Design review of the part built by this model. Coordinates are the model's own, in mm. A direction names the side the tool comes from. Give positions to 0.01 mm unless a question says otherwise; leave off trailing zeros. Loops run counter-clockwise (first coordinate to the right, second up) from the corner with the lowest first, then second, coordinate; pieces in that order, holes last. Notation, with made-up numbers: M 16.5,1.25 L 21.5,1.25 A7 cw 21.5,12.25 Z; hole C 81.25,71.25 d1. An arc over 180 degrees is marked long. Use a Markdown table: item, result. Add a question column.
(1) Draft analysis for pull direction Z (two halves, no side actions). For faces 6 (the face through (-7.5, -19.1, 19.2)), 7 (the face through (-1.404, -15.612, 15.676)), 8 (the face through (-5, -0.1, 20.5)), state which applies: pulls with the +Z half, pulls with the -Z half, needs draft (parallel to the pull), parting line crosses it, or undercut.
(2) Add section D-D, the plane z = 12. Give the boundary of the cut face in (x, y).
(3) Add section C-C, the plane x = 2. Give the boundary of the cut face in (y, z), then the cut area to 3 significant figures.
(4) Insertion check: pin 1 Ø4 at (y, z) = (15.5, 15.5) entering from -X; pin 2 Ø8 at (x, y) = (0, 7) entering from -Z; pin 3 Ø8 at (x, z) = (-0.5, -4.5) entering from +Y. Each pin has a flat end and moves straight along its axis. Give the tip position at first contact, or say it passes through.
(5) For faces 1 (the face through (0, -20.15, 0)), 2 (the face through (8, 0, 21.15)), 3 (the face through (0.07, -18.467, 18.419)), 4 (the face through (8, 0, -21.15)), 5 (the face through (-5.94, 15.24, 14.33)), list the 3-axis set-ups (+Z, -Z, +X, -X, +Y, -Y) from which the entire face can be reached by the end or side of a thin tool; tool diameter is ignored.
(6) For probe 1 along Y at (x, z) = (-4.25, -15.5); probe 2 along Z at (x, y) = (-6.75, 15.5), list the stretches that pass through material, from the lowest coordinate up.
(7) Add section A-A, the plane y = 0. Give the boundary of the cut face in (x, z).
```python
from build123d import *

# Parameters (mm, degrees)
F0_W     = 42.3
F0_H     = 42.3
F1_DEPTH = 10
F2_SIZE  = 4
F3_W     = 43
F3_H     = 43
F4_DEPTH = 5
F5_R     = 2.5
F6_DEPTH = 20
F8_D     = 2.4
F8_DEPTH = 8
F8_TIP   = 0.7210327428


with BuildPart() as f1:
    # F0 (on Right) → F1 (new body, symmetric)
    with BuildSketch(Plane.YZ):
        Rectangle(F0_W, F0_H)
    extrude(amount=F1_DEPTH, both=True)

    # F2
    f2_edges = [f1.edges().sort_by_distance(p)[0] for p in [
        (0, -21.15, 21.15),
        (0, 21.15, 21.15),
        (0, -21.15, -21.15),
        (0, 21.15, -21.15),
    ]]
    chamfer(f2_edges, length=F2_SIZE)

    # F3 (on Right) → F4 (cut, symmetric)
    with BuildSketch(Plane.YZ):
        Rectangle(F3_W, F3_H)
        Polygon((-16.7357864376, -20.15), (-20.15, -16.7357864376), (-20.15, 16.7357864376), (-16.7357864376, 20.15), (16.7357864376, 20.15), (20.15, 16.7357864376), (20.15, -16.7357864376), (16.7357864376, -20.15), align=None, mode=Mode.SUBTRACT)
    extrude(amount=F4_DEPTH, both=True, mode=Mode.SUBTRACT)

    # F5 (on face) → F6 (join)
    with BuildSketch(Plane(origin=(-10, 0, 0), x_dir=(0, -1, 0), z_dir=(-1, 0, 0))):
        Circle(F5_R)
    extrude(amount=F6_DEPTH)

    # F8
    with Locations(Plane(origin=(-10, 0, 0), x_dir=(0, -1, 0), z_dir=(-1, 0, 0))):
        with Locations((-15.5, 15.5), (15.5, 15.5), (-15.5, -15.5), (15.5, -15.5)):
            Hole(F8_D / 2, depth=F8_DEPTH)
            with Locations((0, 0, -(F8_DEPTH + F8_TIP / 2))):  # 118° drill point
                Cone(0, F8_D / 2, F8_TIP, mode=Mode.SUBTRACT)


solid = f1.part
```
Established:
| question | item | result |
|---|---|---|
| 1 | face 6 | pulls with the +Z half |
| 1 | face 7 | undercut |
| 1 | face 8 | needs draft |
| 2 | outline | M -10,-21.15 L -5,-21.15 L -5,-20.15 L 5,-20.15 L 5,-21.15 L 10,-21.15 L 10,21.15 L 5,21.15 L 5,20.15 L -5,20.15 L -5,21.15 L -10,21.15 Z |
| 3 | outline | M -20.15,-16.74 L -16.74,-20.15 L 16.74,-20.15 L 20.15,-16.74 L 20.15,16.74 L 16.74,20.15 L -16.74,20.15 L -20.15,16.74 Z |
| 3 | area | 1,600 mm^2 |
| 4 | pin 1 | x = -10 |
| 4 | pin 2 | z = -20.15 |
| 4 | pin 3 | y = 20.15 |
| 5 | face 1 | +Z, -Z, -Y |
| 5 | face 2 | +Z, +X, -X, +Y, -Y |
| 5 | face 3 | +Z, -Y |
| 5 | face 4 | -Z, +X, -X, +Y, -Y |
| 5 | face 5 | -X |
| 6 | probe 1 | -20.15 to -16.7, -14.3 to 14.3, 16.7 to 20.15 |
| 6 | probe 2 | -21.15 to -16.7, -14.3 to 14.3, 16.7 to 21.15 |
| 7 | outline | M -30,-2.5 L -10,-2.5 L -10,-21.15 L -5,-21.15 L -5,-20.15 L 5,-20.15 L 5,-21.15 L 10,-21.15 L 10,21.15 L 5,21.15 L 5,20.15 L -5,20.15 L -5,21.15 L -10,21.15 L -10,2.5 L -30,2.5 Z |
